Input: dimensioned drawing with shaded views. Units: mm. Origin: part minimum x, y, z. Coordinates: 2 decimals unless noted, no trailing zeros. Order: outer loops, then holes, each group sorted by start corner. A loop starts at its lowest first (then second) coordinate and runs counter-clockwise, first axis right, second up. Notation, with made-up numbers: M -30.5,8.5 L 19.5,8.5 A21 cw 19.5,39.5 Z; hole C 7,86 d9. An arc over 180 degrees is marked long. Write item = value, one per line.
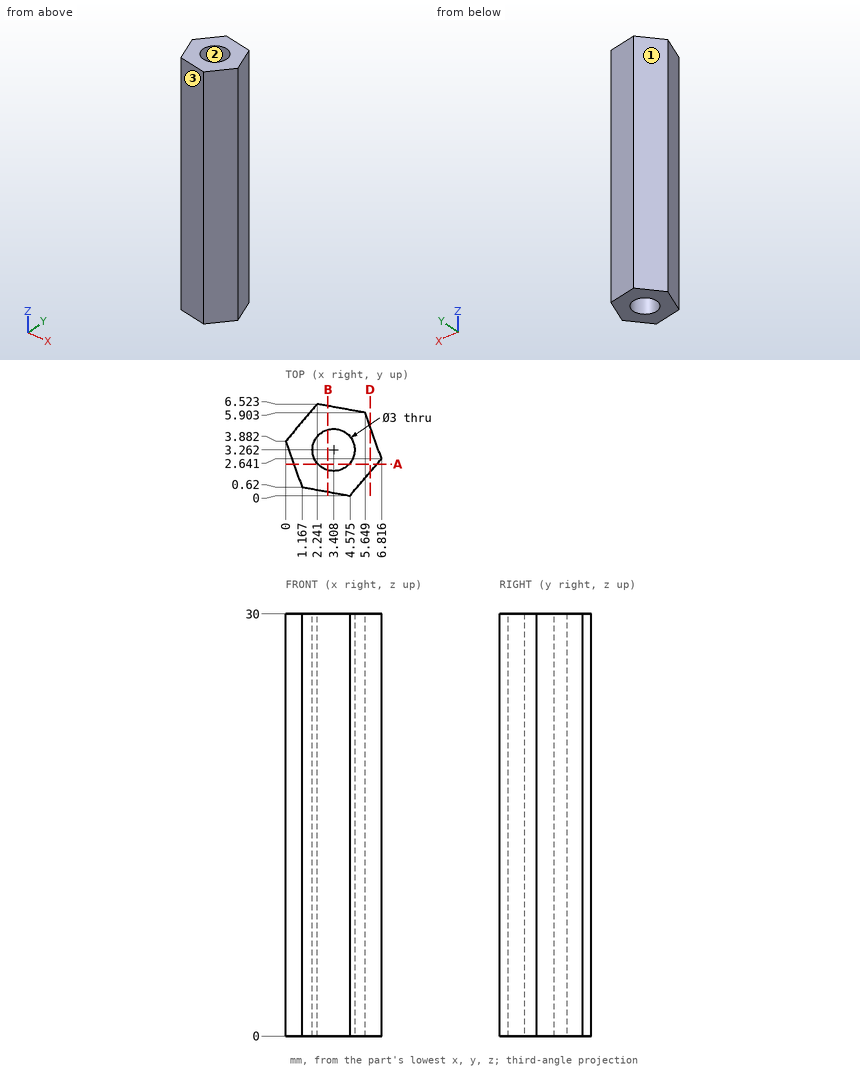
1) Section D-D, the plane x = 6. Return loops of the section in (y, z).
Numbers:
outline = M 1.68,0 L 4.92,0 L 4.92,30 L 1.68,30 Z
2) Section A-A, the plane y = 2.25. Return loops of the section in (x, z) (1 decimal).
Numbers:
outline = M 0.6,0 L 2.3,0 L 2.3,30 L 0.6,30 Z; M 4.5,0 L 6.5,0 L 6.5,30 L 4.5,30 Z
3) Pin query (flat end, axial travel): pin 1 (1.5 mm diameter, centred on y = 4.5, z = 20.5, fed in from +X); pin 2 (2 mm diameter, centred on x = 6, z = 24.5, fed in from -Y). Return the tip coordinate at first contact, or that it passes through.
Numbers:
pin_1 = 6.42
pin_2 = 0.5
4) Section B-B, the plane x = 3. Return loops of the section in (y, z) (1 decimal).
Numbers:
outline = M 0.3,0 L 1.8,0 L 1.8,30 L 0.3,30 Z; M 4.7,0 L 6.4,0 L 6.4,30 L 4.7,30 Z
5) Line query: L1, parallel to X at y = 4.25, z = 17.75 (1 decimal); L2, parallel to X at y = 3.5, z = 26.5; L3, parallel to Y at x = 3, z = 9.5 (1 decimal). Output: solid intervals per line, ascending.
Numbers:
L1 = 0.3 to 2.3, 4.5 to 6.2
L2 = 0.14 to 1.93, 4.89 to 6.51
L3 = 0.3 to 1.8, 4.7 to 6.4
6) Mould query, pull axis Y, two halves, no side actions, for the marked faces 1, 2 and 3. Classes: pulls with the +Y half, pulls with the -Y half, needs draft (parallel to the pull), parting line crosses it, or undercut.
Numbers:
face_1 = pulls with the +Y half
face_2 = undercut
face_3 = pulls with the -Y half
